```python
from build123d import *

# Parameters (mm, degrees)
SKETCH_1_W          = 68
SKETCH_1_H          = 35
SKETCH_1_R          = 1.5
EXTRUDE_1_DEPTH     = 4
FILLET_1_R          = 3
SKETCH_2_R          = 1.5
SKETCH_2_R_2        = 7.5
CUT_EXTRUDE_1_DEPTH = 10


with BuildPart() as part:
    # 草图1 → 凸台-拉伸1 (new body)
    with BuildSketch(Plane(origin=(0, 0, 0), x_dir=(1, 0, 0), z_dir=(0, 1, 0))):
        Rectangle(SKETCH_1_W, SKETCH_1_H)
        with Locations(Location((-30, 12.5, 0), (0, 0, 270))):
            Circle(SKETCH_1_R, mode=Mode.SUBTRACT)
        with Locations(Location((-30, 4.5, 0), (0, 0, 270))):
            Circle(SKETCH_1_R, mode=Mode.SUBTRACT)
        with Locations(Location((-30, -5.5, 0), (0, 0, 270))):
            Circle(SKETCH_1_R, mode=Mode.SUBTRACT)
        with Locations(Location((-30, -13.5, 0), (0, 0, 270))):
            Circle(SKETCH_1_R, mode=Mode.SUBTRACT)
    extrude(amount=EXTRUDE_1_DEPTH)

    # 圆角1
    fillet_1_edges = [part.edges().sort_by_distance(p)[0] for p in [
        (34, 2, 17.5),
        (-34, 2, 17.5),
        (-34, 2, -17.5),
        (34, 2, -17.5),
    ]]
    fillet(fillet_1_edges, radius=FILLET_1_R)

    # 草图2 → 切除-拉伸1 (cut)
    with BuildSketch(Plane(origin=(0, 4, 0), x_dir=(1, 0, 0), z_dir=(0, 1, 0))):
        with Locations(Location((-21, 0.5, 0), (0, 0, 270))):
            Circle(SKETCH_2_R)
        with Locations(Location((30, 0.5, 0), (0, 0, 270))):
            Circle(SKETCH_2_R)
        with Locations(Location((-21, -9.5, 0), (0, 0, 270))):
            Circle(SKETCH_2_R)
        with Locations(Location((30, -9.5, 0), (0, 0, 270))):
            Circle(SKETCH_2_R)
        with Locations(Location((5, 0, 0), (0, 0, 270))):
            Circle(SKETCH_2_R_2)
    extrude(amount=-CUT_EXTRUDE_1_DEPTH, mode=Mode.SUBTRACT)


solid = part.part
```
Geometry check sheet. Reference: the model listing, model coordinates, mm. Round coordinates to 2 decimals unless told otherwise and drop trailing zeros. Order: outer loops, then holes, each group sorted by start corner. A loop starts at its lowest first (then second) coordinate and runs counter-clockwise, first axis right, second up. Notation, with made-up numbers: M 67,-16.75 L 88,-16.75 A14 cw 88,-5.75 Z; hole C 19.5,-14 d3. An arc over 180 degrees is marked long. Answer as CSV lines item,"result".
1) Sectioned sample at A-A on x = -30. Record the cut outline in (y, z), and give its area (3 significant figures).
Entries:
outline,"M 0,-17.5 L 4,-17.5 L 4,-14 L 0,-14 Z; M 0,-11 L 4,-11 L 4,-6 L 0,-6 Z; M 0,-3 L 4,-3 L 4,4 L 0,4 Z; M 0,7 L 4,7 L 4,12 L 0,12 Z; M 0,15 L 4,15 L 4,17.5 L 0,17.5 Z"
area,"92.0 mm2"
2) Sectioned sample at B-B on z = -12.5. Record the cut outline in (x, y).
Entries:
outline,"M -34,0 L -31.5,0 L -31.5,4 L -34,4 Z; M -28.5,0 L 34,0 L 34,4 L -28.5,4 Z"
3) Gauge pin test, flat end, axial feed: pin 1 Ø2.5 at (x, z) = (-21, -0.5) entering from -Y. Record the tip position at first contact, or that the pin passes through.
Entries:
pin 1,"through"
4) Mould release check, pull along X, two halves, no side actions. Record for faces 1 (the face through (-33.14, 2.03, 16.6)), 2 (the face through (33.1, 2.03, 16.64)), 3 (the face through (-28.513, 1.972, -4.695)): +X half, -X half, draft (parallel to the pull), parting line (faces both ways), or undercut.
Entries:
face 1,"-X half"
face 2,"+X half"
face 3,"undercut"
5) Thickness scan on probe 1 along X at (y, z) = (1.35, 9.5); probe 2 along X at (y, z) = (3.2, -12.5); probe 3 along X at (y, z) = (3.6, -4.5). Record the ranges inside material, lowest first. Write a range as [from, to].
Entries:
probe 1,"[-34, -22.5], [-19.5, 28.5], [31.5, 34]"
probe 2,"[-34, -31.5], [-28.5, 34]"
probe 3,"[-34, -31.5], [-28.5, -1], [11, 34]"
6) Sectioned sample at D-D on x = -21. Record the cut outline in (y, z), and give its area (3 significant figures).
Entries:
outline,"M 0,-17.5 L 4,-17.5 L 4,-2 L 0,-2 Z; M 0,1 L 4,1 L 4,8 L 0,8 Z; M 0,11 L 4,11 L 4,17.5 L 0,17.5 Z"
area,"116 mm2"
7) Sectioned sample at C-C on y = 3. Give the number of separate pieces and of enclosed holes in the cut face, and give its area (3 significant figures).
Entries:
separate pieces,"1"
enclosed holes,"9"
area,"2,140 mm2"
